Autodesk Inventor part; units mm, degrees
ref_plane "YZ Plane" through (0, 0, 0) normal (1, 0, 0) x (0, 1, 0)
ref_plane "XZ Plane" through (0, 0, 0) normal (0, 1, 0) x (-1, 0, 0)
ref_plane "XY Plane" through (0, 0, 0) normal (0, 0, 1) x (1, 0, 0)
sketch "Sketch1" plane through (0, 0, 0) normal (0, 0, 1) x (1, 0, 0)
  line L0 (63.5, 50.8) -> (63.5, 44.45)
  circle A0 centre (63.5, 44.45) radius 38.1
  circle A1 centre (33.655, 74.295) radius 2.1082
  circle A2 centre (93.345, 74.295) radius 2.1082
  circle A3 centre (93.345, 14.605) radius 2.1082
  circle A4 centre (33.655, 14.605) radius 2.1082
  line L1 (63.5, 82.55) -> (63.5, 86.36)
  line L2 (63.5, 86.36) -> (82.55, 86.36)
  line L3 (63.5, 86.36) -> (44.45, 86.36)
  line L4 (82.55, 86.36) -> (82.55, 134.62)
  line L5 (44.45, 86.36) -> (44.45, 134.62)
  arc A5 (82.55, 134.62) -> (44.45, 134.62) centre (63.5, 134.62) ccw
  arc A6 (-2.400661, 17.597517) -> (12.7, -3.175) centre (12.7, 12.7) ccw
  arc A7 (114.3, -3.175) -> (129.400661, 17.597517) centre (114.3, 12.7) ccw
  line L6 (114.3, -3.175) -> (12.7, -3.175)
  line L7 (48.399339, 174.230681) -> (-2.400661, 17.597517)
  line L8 (129.400661, 17.597517) -> (78.600661, 174.230681)
  arc A8 (78.600661, 174.230681) -> (48.399339, 174.230681) centre (63.5, 169.333164) ccw
  arc A9 (75.580529, 173.251177) -> (51.419471, 173.251177) centre (63.5, 169.333164) ccw
  arc A10 (0.619471, 16.618013) -> (12.7, 0) centre (12.7, 12.7) ccw
  arc A11 (114.3, 0) -> (126.380529, 16.618013) centre (114.3, 12.7) ccw
  line L9 (12.7, 0) -> (114.3, 0)
  line L10 (0.619471, 16.618013) -> (51.419471, 173.251177)
  line L11 (75.580529, 173.251177) -> (126.380529, 16.618013)
  line L12 (0.619471, 16.618013) -> (3.753882, 26.282436)
  line L13 (3.753882, 26.282436) -> (4.961935, 25.890635)
  circle A12 centre (4.961935, 25.890635) radius 1.27
  line L14 (51.419471, 173.251177) -> (48.285061, 163.586755)
  line L15 (48.285061, 163.586755) -> (49.493113, 163.194953)
  circle A13 centre (49.493113, 163.194953) radius 1.27
  circle A14 centre (27.227524, 94.542794) radius 1.27
  line L16 (75.580529, 173.251177) -> (78.714939, 163.586755)
  line L17 (78.714939, 163.586755) -> (77.506886, 163.194953)
  circle A15 centre (77.506886, 163.194953) radius 1.27
  line L18 (126.380529, 16.618013) -> (123.246118, 26.282436)
  line L19 (123.246118, 26.282436) -> (122.038065, 25.890635)
  circle A16 centre (122.038065, 25.890635) radius 1.27
  circle A17 centre (99.772476, 94.542794) radius 1.27
  line L20 (12.7, 0) -> (16.51, 0)
  line L21 (18.621315, -3.175) -> (18.621315, 1.27) construction
  line L22 (45.72, 1.27) -> (50.8, 1.27) construction
  line L23 (12.7, 0.808162) -> (16.51, 0.808162) construction
  circle A18 centre (50.8, 1.27) radius 1.27
  line L24 (109.391635, -3.175) -> (109.391635, 1.27) construction
  line L25 (81.28, 1.27) -> (76.2, 1.27) construction
  line L26 (114.432893, 0.578481) -> (110.622893, 0.578481) construction
  circle A19 centre (76.2, 1.27) radius 1.27
  point P0 (0, 0)
  point P1 (0, 0)
  dimension "d13" = 76.2
  dimension "d42" = 2.54
  dimension "d45" = 2.54
  dimension "d12" = 6.35
  dimension "d14" = 4.2164
  dimension "d15" = 4.2164
  dimension "d16" = 4.2164
  dimension "d17" = 4.2164
  dimension "d18" = 3.81
  dimension "d19" = 19.05
  dimension "d20" = 19.05
  dimension "d21" = 48.26
  dimension "d22" = 48.26
  dimension "d26" = 31.75
  dimension "d27" = 31.75
  dimension "d30" = 25.4
  dimension "d31" = 25.4
  dimension "d32" = 25.4
  dimension "d33" = 10.16
  dimension "d34" = 10.16
  dimension "d35" = 1.27
  dimension "d37" = 1.27
  dimension "d40" = 10.16
  dimension "d41" = 10.16
  dimension "d43" = 2.54
  dimension "d44" = 2.54
  dimension "d221" = 4.445
  dimension "d222" = 5.08
  dimension "d224" = 5.08
  dimension "d225" = 3.81
  dimension "d228" = 38.1
  dimension "d229" = 38.1
sketch "Sketch1 outline for Extrusion3" plane through (0, 0, 0) normal (0, 0, 1) x (1, 0, 0)
  arc A0 (78.600661, 174.230681) -> (48.399339, 174.230681) centre (63.5, 169.333164) ccw
  line L0 (129.400661, 17.597517) -> (78.600661, 174.230681)
  line L1 (48.399339, 174.230681) -> (-2.400661, 17.597517)
  arc A1 (114.3, -3.175) -> (129.400661, 17.597517) centre (114.3, 12.7) ccw
  arc A2 (-2.400661, 17.597517) -> (12.7, -3.175) centre (12.7, 12.7) ccw
  line L2 (12.7, -3.175) -> (114.3, -3.175)
  circle A3 centre (4.961935, 25.890635) radius 1.27
  circle A4 centre (33.655, 14.605) radius 2.1082
  circle A5 centre (33.655, 74.295) radius 2.1082
  circle A6 centre (93.345, 14.605) radius 2.1082
  circle A7 centre (63.5, 44.45) radius 38.1
  circle A8 centre (122.038065, 25.890635) radius 1.27
  circle A9 centre (93.345, 74.295) radius 2.1082
  circle A10 centre (27.227524, 94.542794) radius 1.27
  circle A11 centre (49.493113, 163.194953) radius 1.27
  line L3 (44.45, 86.36) -> (63.5, 86.36)
  line L4 (63.5, 86.36) -> (82.55, 86.36)
  line L5 (82.55, 86.36) -> (82.55, 134.62)
  arc A12 (82.55, 134.62) -> (44.45, 134.62) centre (63.5, 134.62) ccw
  line L6 (44.45, 134.62) -> (44.45, 86.36)
  circle A13 centre (99.772476, 94.542794) radius 1.27
  circle A14 centre (77.506886, 163.194953) radius 1.27
extrude "Extrusion3" add sketch "Sketch1 outline for Extrusion3" along normal blind 4.572
sketch "Sketch2" plane through (0, 0, 4.572) normal (0, 0, 1) x (1, 0, 0)
  line L0 (44.45, 86.36) -> (82.55, 86.36)
  line L1 (63.5, 86.36) -> (44.45, 86.36)
  line L2 (63.5, 86.36) -> (82.55, 86.36)
  line L3 (53.975, 86.36) -> (63.5, 86.36)
  line L4 (63.5, 86.36) -> (73.025, 86.36)
  line L5 (82.55, 134.62) -> (82.55, 86.36)
  line L6 (71.882, 140.7922) -> (76.962, 140.7922)
  line L7 (76.962, 140.7922) -> (76.962, 89.9922)
  line L8 (76.962, 89.9922) -> (71.882, 89.9922)
  line L9 (71.882, 89.9922) -> (71.882, 140.7922)
  circle A0 centre (70.07225, 128.0922) radius 1.3335
  circle A1 centre (70.07225, 102.6922) radius 1.3335
  line L10 (50.038, 89.9922) -> (55.118, 89.9922)
  line L11 (55.118, 89.9922) -> (55.118, 140.7922)
  line L12 (55.118, 140.7922) -> (50.038, 140.7922)
  line L13 (50.038, 140.7922) -> (50.038, 89.9922)
  line L14 (44.45, 86.36) -> (44.45, 134.62)
  circle A2 centre (48.22825, 128.0922) radius 1.3335
  circle A3 centre (48.22825, 102.6922) radius 1.3335
  line L15 (71.882, 99.06) -> (68.73875, 99.06)
  line L16 (66.04, 99.06) -> (60.96, 99.06)
  line L17 (60.96, 99.06) -> (60.96, 149.86)
  line L18 (60.96, 149.86) -> (66.04, 149.86)
  line L19 (66.04, 149.86) -> (66.04, 99.06)
  circle A4 centre (59.15025, 111.76) radius 1.3335
  circle A5 centre (59.15025, 137.16) radius 1.3335
  arc A6 (82.55, 134.62) -> (44.45, 134.62) centre (63.5, 134.62) ccw
  line L20 (44.45, 134.62) -> (44.45, 86.36)
  point P0 (0, 0)
  dimension "d183" = 5.08
  dimension "d184" = 50.8
  dimension "d185" = 3.6322
  dimension "d186" = 5.588
  dimension "d189" = 2.667
  dimension "d194" = 5.08
  dimension "d196" = 3.6322
  dimension "d197" = 5.588
  dimension "d198" = 50.8
  dimension "d199" = 1.80975
  dimension "d203" = 2.667
  dimension "d204" = 2.667
  dimension "d205" = 1.80975
  dimension "d207" = 41.7322
  dimension "d208" = 16.3322
  dimension "d209" = 1.80975
  dimension "d211" = 5.08
  dimension "d212" = 50.8
  dimension "d216" = 2.667
  dimension "d217" = 2.667
extrude "Extrusion11" add sketch "Sketch2" against normal blind 4.572
sketch "Sketch3" plane through (0, 0, 4.572) normal (0, 0, 1) x (1, 0, 0)
  point P0 (0, 0)
sketch "Sketch1 outline for Extrusion12" plane through (0, 0, 0) normal (0, 0, 1) x (1, 0, 0)
  circle A0 centre (50.8, 1.27) radius 1.27
  circle A1 centre (76.2, 1.27) radius 1.27
extrude "Extrusion12" cut sketch "Sketch1 outline for Extrusion12" along normal blind 4.572
properties part number "Nathan_LED_Speaker_Front"
Geometry check sheet. Reference: the model listing, model coordinates, mm. A direction names the side the tool comes from. Coordinates: 2 decimals unless noted, no trailing zeros. Write each loop counter-clockwise with the first axis right and the second up, starting at its lowest first coordinate (ties: lowest second). Pieces come first, ordered by that corner, then holes. Notation, with made-up numbers: (19, 51.5) -> (31, 51.5) arc R13 ccw to (31, 73.5) -> close; hole circle Ø9 at (-22.5, 32). An arc over 180 degrees is marked (long way). Use CSV: the item, a comma, the result in double quotes. Start each with the question number.
Item 1: Mould release check, pull along X, two halves, no side actions. Record for faces 1 (the flat face through (63, 92, 0)), 2 (the cylindrical face through (91.672, 15.888, 2.254)), 3 (the flat face through (104.356, 94.818, 2.254)), 4 (the flat face through (71.882, 115, 2)): released by +X, released by -X, zero draft, split by the parting line, or undercut.
Item 2: Cross-section at D-D, the plane z = 1.5. State how many separate pieces and enclosed holes the cut face has, plus the area to 3 significant figures.
Item 3: Set-up check for faces 5 (the flat face through (50.038, 116, 2)), 6 (the flat face through (63, 92, 4.572)): record each of +Z, -Z, +X, -X, +Y, -Y from which the full face is reachable in a straight line by a thin tool's end or side.
Item 4: Cross-section at A-A, the plane x = 63.5. Record the cut outline in (y, z) (3 decimals), plus the area to 3 significant figures.
Item 5: Cross-section at C-C, the plane y = 106.5. Record the cut outline in (x, z).
Item 6: Cross-section at B-B, the plane y = 64. Record the cut outline in (x, z).
Item 7: Depth check by flat-ended pin: pin 1 Ø2.5 at (y, z) = (114.5, 1.5) entering from -X; pin 2 Ø1.5 at (x, y) = (76.2, 1.27) entering from -Z; pin 3 Ø1.4 at (x, z) = (73.5, 2) entering from +Y. Enter the tip coordinate at first touch or a pass-through.
Item 8: Thickness scan on line 1 (X direction, y = 105, z = 2.85); line 2 (Y direction, x = 63.5, z = 2.3) (3 decimals); line 3 (X direction, y = 137, z = 1.25). Record the ranges inside material, lowest first.
Answers:
1,face 1,"zero draft"
1,face 2,"undercut"
1,face 3,"released by +X"
1,face 4,"undercut"
2,separate pieces,"1"
2,enclosed holes,"22"
2,area,"10,100 mm^2"
3,face 5,"+Z, -Z"
3,face 6,"+Z, +X, -X, +Y, -Y"
4,outline,"(-3.175, 0) -> (6.35, 0) -> (6.35, 4.572) -> (-3.175, 4.572) -> close; (82.55, 0) -> (99.06, 0) -> (99.06, 4.572) -> (82.55, 4.572) -> close; (149.86, 0) -> (185.208, 0) -> (185.208, 4.572) -> (149.86, 4.572) -> close"
4,area,"281 mm^2"
5,outline,"(26.43, 0) -> (50.04, 0) -> (50.04, 4.57) -> (26.43, 4.57) -> close; (55.12, 0) -> (60.96, 0) -> (60.96, 4.57) -> (55.12, 4.57) -> close; (66.04, 0) -> (71.88, 0) -> (71.88, 4.57) -> (66.04, 4.57) -> close; (76.96, 0) -> (100.57, 0) -> (100.57, 4.57) -> (76.96, 4.57) -> close"
6,outline,"(12.65, 0) -> (30.8, 0) -> (30.8, 4.57) -> (12.65, 4.57) -> close; (96.2, 0) -> (114.35, 0) -> (114.35, 4.57) -> (96.2, 4.57) -> close"
7,pin 1,"x = 28.62"
7,pin 2,"through"
7,pin 3,"y = 182.2"
8,line 1,"25.95 to 50.04, 55.12 to 60.96, 66.04 to 71.88, 76.96 to 101.05"
8,line 2,"-3.175 to 6.35, 82.55 to 99.06, 149.86 to 185.208"
8,line 3,"36.32 to 50.04, 55.12 to 57.83, 60.47 to 60.96, 66.04 to 71.88, 76.96 to 90.68"
